Check sheet for the modelled part. Datum: model origin and axes. Units: mm. Face numbers are marked on the shaded views. Round coordinates to 2 decimals unless told otherwise and drop trailing zeros. Order: outer loops, then holes, each group sorted by start corner. A loop starts at its lowest first (then second) coordinate and runs counter-clockwise, first axis right, second up. Notation, with made-up numbers: (-26.5, -13) -> (8.5, -13) arc R37 ccw to (8.5, 23) -> close; hole circle Ø9 at (-26, -1). An arc over 180 degrees is marked (long way). Answer in a Markdown table with one row per item.
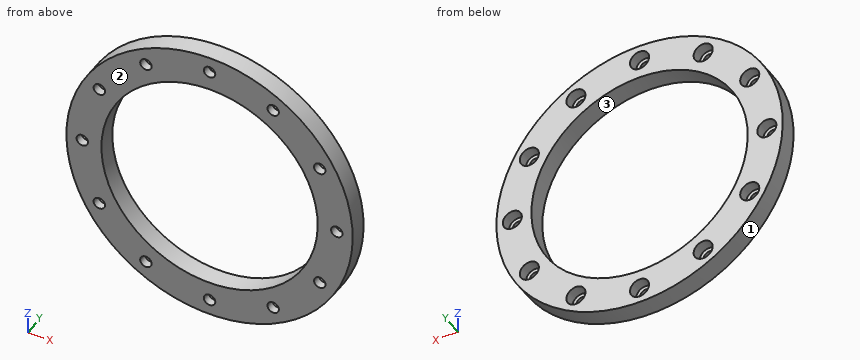
from build123d import *

# Parameters (mm, degrees)
SKETCH_1_R                = 45
SKETCH_1_R_2              = 34
EXTRUDE_1_DEPTH           = 6
HOLE_WIZARD_1_D           = 3.6
HOLE_WIZARD_1_CBORE_D     = 6
HOLE_WIZARD_1_CBORE_DEPTH = 3.4
PATTERN_CIRCULAR_1_COUNT  = 12


with BuildPart() as part:
    # Sketch 1 → Extrude 1 (new body)
    with BuildSketch(Plane(origin=(0, 0, 0), x_dir=(1, 0, 0), z_dir=(0, 1, 0))):
        with Locations(Location((0, 0, 0), (0, 0, 270))):
            Circle(SKETCH_1_R)
        with Locations(Location((0, 0, 0), (0, 0, 270))):
            Circle(SKETCH_1_R_2, mode=Mode.SUBTRACT)
    extrude(amount=EXTRUDE_1_DEPTH)

    # Hole Wizard 1 (through all)
    with Locations(Plane(origin=(0, 6, 0), x_dir=(1, 0, 0), z_dir=(0, 1, 0))):
        with Locations((0, 40)):
            hole_wizard_1 = CounterBoreHole(HOLE_WIZARD_1_D / 2, HOLE_WIZARD_1_CBORE_D / 2, HOLE_WIZARD_1_CBORE_DEPTH)

    # Pattern Circular 1: Hole Wizard 1 ×12 about axis
    pattern_circular_1_axis = Axis((0, 0, 0), (0, 1, 0))
    for i in range(1, PATTERN_CIRCULAR_1_COUNT):
        add(hole_wizard_1.rotate(pattern_circular_1_axis, i * 360 / PATTERN_CIRCULAR_1_COUNT), mode=Mode.SUBTRACT)


solid = part.part
Item 1: Cross-section at B-B (x = 20). Record the boundary of the cut face in (y, z).
Result sheet:
| item | result |
|---|---|
| outline | (0, -40.31) -> (6, -40.31) -> (6, -37.64) -> (2.6, -37.64) -> (2.6, -36.44) -> (0, -36.44) -> close; (0, -32.84) -> (2.6, -32.84) -> (2.6, -31.64) -> (6, -31.64) -> (6, -27.5) -> (0, -27.5) -> close; (0, 27.5) -> (6, 27.5) -> (6, 31.64) -> (2.6, 31.64) -> (2.6, 32.84) -> (0, 32.84) -> close; (0, 36.44) -> (2.6, 36.44) -> (2.6, 37.64) -> (6, 37.64) -> (6, 40.31) -> (0, 40.31) -> close |
Item 2: Scan lines: line 1 (X direction, y = 4.3, z = 0); line 2 (Z direction, x = 34.5, y = 0.3); line 3 (X direction, y = 3.45, z = 35). Record each from-to range of solid material in increasing order. Write a range as [from, to].
Result sheet:
| item | result |
|---|---|
| line 1 | x = [-45, -43], [-37, -34], [34, 37], [43, 45] |
| line 2 | z = [-28.89, -21.79], [-18.21, 18.21], [21.79, 28.89] |
| line 3 | x = [-28.28, -22.98], [-17.02, 17.02], [22.98, 28.28] |
Item 3: Depth check by flat-ended pin: P1, Ø9.5, axis at x = 40, z = 0, coming from the +Y side; P2, Ø3, axis at x = 33.5, z = -19.5, coming from the +Y side; P3, Ø1.5, axis at x = 19.5, y = 4.5, coming from the +Z side; P4, Ø1.5, axis at y = 4, z = -35.5, coming from the -X side. Enter the tip coordinate at first touch or a pass-through.
Result sheet:
| item | result |
|---|---|
| P1 | stops at y = 6 |
| P2 | stops at y = 2.6 |
| P3 | stops at z = 40.91 |
| P4 | stops at x = -28.59 |
Item 4: Mould release check, pull along Z, two halves, no side actions. Record for the marked faces 1, 2 and 3: pulls with the +Z half, pulls with the -Z half, needs draft (parallel to the pull), parting line crosses it, or undercut.
Result sheet:
| item | result |
|---|---|
| face 1 | parting line crosses it |
| face 2 | needs draft |
| face 3 | undercut |
Item 5: Cross-section at A-A (z = 0). Record the boundary of the cut face in (x, y), and give its area (3 significant figures).
Result sheet:
| item | result |
|---|---|
| outline | (-45, 0) -> (-41.8, 0) -> (-41.8, 2.6) -> (-43, 2.6) -> (-43, 6) -> (-45, 6) -> close; (-38.2, 0) -> (-34, 0) -> (-34, 6) -> (-37, 6) -> (-37, 2.6) -> (-38.2, 2.6) -> close; (34, 0) -> (38.2, 0) -> (38.2, 2.6) -> (37, 2.6) -> (37, 6) -> (34, 6) -> close; (41.8, 0) -> (45, 0) -> (45, 6) -> (43, 6) -> (43, 2.6) -> (41.8, 2.6) -> close |
| area | 72.5 mm^2 |
Item 6: Cross-section at C-C (z = -40). Record the boundary of the cut face in (x, y), and give its area (3 significant figures).
Result sheet:
| item | result |
|---|---|
| outline | (-20.62, 0) -> (-1.8, 0) -> (-1.8, 2.6) -> (-3, 2.6) -> (-3, 6) -> (-20.62, 6) -> close; (1.8, 0) -> (20.62, 0) -> (20.62, 6) -> (3, 6) -> (3, 2.6) -> (1.8, 2.6) -> close |
| area | 218 mm^2 |
Item 7: Cross-section at D-D (x = 40). Record the boundary of the cut face in (y, z).
Result sheet:
| item | result |
|---|---|
| outline | (0, -20.62) -> (6, -20.62) -> (6, -3) -> (2.6, -3) -> (2.6, -1.8) -> (0, -1.8) -> close; (0, 1.8) -> (2.6, 1.8) -> (2.6, 3) -> (6, 3) -> (6, 20.62) -> (0, 20.62) -> close |
